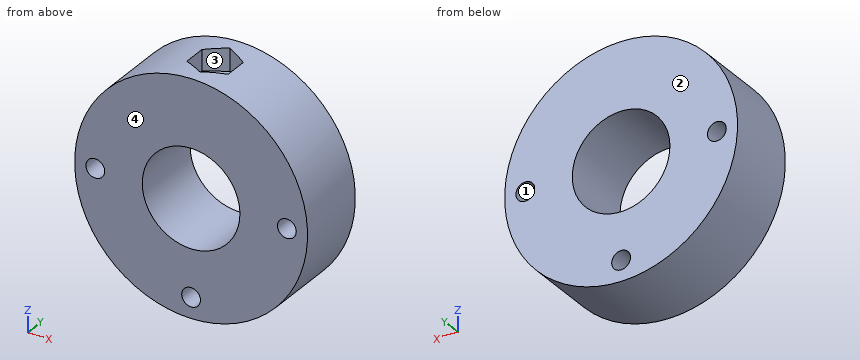
```python
from build123d import *

# Parameters (mm, degrees)
SKETCH1_R           = 31
SKETCH1_R_2         = 13
SKETCH1_R_3         = 2.5
BOSS_EXTRUDE1_DEPTH = 20
CUT_EXTRUDE1_DEPTH  = 15


with BuildPart() as part:
    # Sketch1 → Boss-Extrude1 (new body)
    with BuildSketch(Plane(origin=(0, 0, 0), x_dir=(1, 0, 0), z_dir=(0, 1, 0))):
        with Locations(Location((0, 0, 0), (0, 0, 270))):
            Circle(SKETCH1_R)
        with Locations(Location((0, 0, 0), (0, 0, 270))):
            Circle(SKETCH1_R_2, mode=Mode.SUBTRACT)
        with Locations(Location((0, 25.5, 0), (0, 0, 270))):
            Circle(SKETCH1_R_3, mode=Mode.SUBTRACT)
        with Locations(Location((-25.5, 0, 0), (0, 0, 270))):
            Circle(SKETCH1_R_3, mode=Mode.SUBTRACT)
        with Locations(Location((25.5, 0, 0), (0, 0, 270))):
            Circle(SKETCH1_R_3, mode=Mode.SUBTRACT)
    extrude(amount=BOSS_EXTRUDE1_DEPTH)

    # Sketch3 → Cut-Extrude1 (cut)
    with BuildSketch(Plane.XY.offset(40)):
        Polygon((-5.5, 6.824573519), (0, 3.649147039), (5.5, 6.824573519), (5.5, 13.175426481), (0, 16.350852961), (-5.5, 13.175426481), align=None)
    extrude(amount=-CUT_EXTRUDE1_DEPTH, mode=Mode.SUBTRACT)


solid = part.part
```
Check sheet for the modelled part. Datum: model origin and axes. Units: mm. Face numbers are marked on the shaded views. Coordinates: 2 decimals unless noted, no trailing zeros. Write each loop counter-clockwise with the first axis right and the second up, starting at its lowest first coordinate (ties: lowest second). Pieces come first, ordered by that corner, then holes. Notation, with made-up numbers: M -5.5,20 L 46.5,20 A5 ccw 46.5,29 Z; hole C 77,1.25 d9. An arc over 180 degrees is marked long. Write item = value, one per line. Start each with the question number.
1. Thickness scan on probe 1 along X at (y, z) = (6.75, 0); probe 2 along X at (y, z) = (18.5, 6); probe 3 along X at (y, z) = (12.25, -25.5). Record the ranges inside material, lowest first.
2. Mould release check, pull along Y, two halves, no side actions. Record for the marked faces 1, 2, 3 and 4: pulls with the +Y half, pulls with the -Y half, needs draft (parallel to the pull), parting line crosses it, or undercut.
3. Sectioned sample at D-D (z = -25.5). Record the cut outline in (x, y).
4. Go/stop test with flat-tipped pins: pin 1 (2 mm diameter, centred on y = 7, z = -23.5, fed in from +X); pin 2 (2 mm diameter, centred on y = 9.5, z = 1, fed in from -X); pin 3 (2 mm diameter, centred on y = 8, z = -1.5, fed in from +X); pin 4 (6.5 mm diameter, centred on x = 0, z = -25.5, fed in from +Y). Record where each tip stops, or that it passes through.
5. Sectioned sample at A-A (z = 0). Record the cut outline in (x, y).
6. Sectioned sample at B-B (x = -25.5). Record the cut outline in (y, z), then the cut area to 3 significant figures.
7. Sectioned sample at C-C (y = 7.75). Record the cut outline in (x, z).
The answers:
q1.probe_1 = -31 to -28, -23 to -13, 13 to 23, 28 to 31
q1.probe_2 = -30.41 to -11.53, 11.53 to 30.41
q1.probe_3 = -17.63 to -2.5, 2.5 to 17.63
q2.face_1 = needs draft
q2.face_2 = pulls with the +Y half
q2.face_3 = undercut
q2.face_4 = pulls with the -Y half
q3.outline = M -17.63,0 L -2.5,0 L -2.5,20 L -17.63,20 Z; M 2.5,0 L 17.63,0 L 17.63,20 L 2.5,20 Z
q4.pin_1 = 21.32
q4.pin_2 = -31
q4.pin_3 = 31
q4.pin_4 = 20
q5.outline = M -31,0 L -28,0 L -28,20 L -31,20 Z; M -23,0 L -13,0 L -13,20 L -23,20 Z; M 13,0 L 23,0 L 23,20 L 13,20 Z; M 28,0 L 31,0 L 31,20 L 28,20 Z
q6.outline = M 0,-17.63 L 20,-17.63 L 20,-2.5 L 0,-2.5 Z; M 0,2.5 L 20,2.5 L 20,17.63 L 0,17.63 Z
q6.area = 605 mm²
q7.outline = M -5.5,25 L -5.5,30.51 A31 ccw long 5.5,30.51 L 5.5,25 Z; hole C -25.5,0 d5; hole C 0,0 d26; hole C 0,-25.5 d5; hole C 25.5,0 d5
